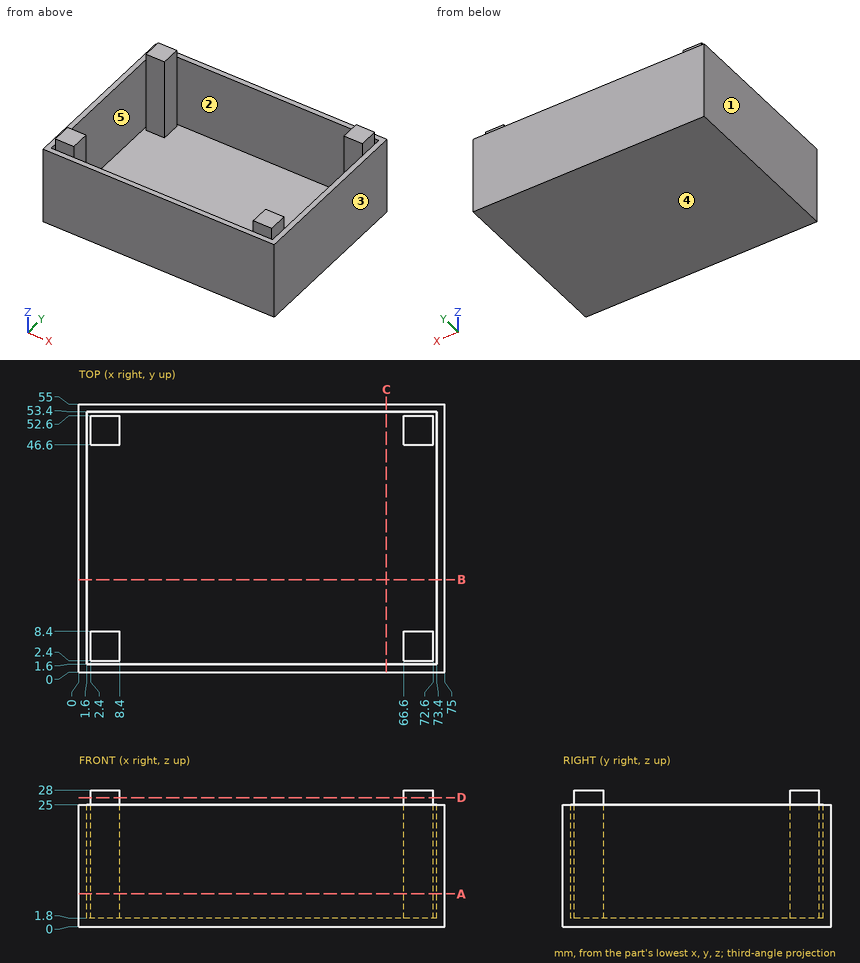
Check sheet for the drawn part. Datum: minimum x, y, z corner. Units: mm. A direction names the side the tool comes from. Give positions to 0.01 mm unless a question says otherwise; leave off trailing zeros. Write each loop counter-clockwise with the first axis right and the second up, starting at its lowest first coordinate (ties: lowest second). Pieces come first, ordered by that corner, then holes. Notation, with made-up numbers: M 54,12.25 L 80,12.25 A19 ccw 80,40.25 Z; hole C 18.25,35 d5. An arc over 180 degrees is marked long. Write item = value, one per line.
(1) Sectioned sample at D-D (z = 26.5). Record the cut outline in (x, y), then the cut area to 3 significant figures.
Found:
outline = M 2.4,2.4 L 8.4,2.4 L 8.4,8.4 L 2.4,8.4 Z; M 2.4,46.6 L 8.4,46.6 L 8.4,52.6 L 2.4,52.6 Z; M 66.6,2.4 L 72.6,2.4 L 72.6,8.4 L 66.6,8.4 Z; M 66.6,46.6 L 72.6,46.6 L 72.6,52.6 L 66.6,52.6 Z
area = 144 mm2
(2) Draft check along X on the marked faces 1, 2 and 3. Enter one of: released by +X, released by -X, zero draft, split by the parting line, or undercut.
Found:
face_1 = released by -X
face_2 = undercut
face_3 = released by +X
(3) Sectioned sample at B-B (y = 19). Record the cut outline in (x, z), then the cut area to 3 significant figures.
Found:
outline = M 0,0 L 75,0 L 75,25 L 73.4,25 L 73.4,1.8 L 1.6,1.8 L 1.6,25 L 0,25 Z
area = 209 mm2
(4) Go/stop test with a flat-tipped pin: pin 1 Ø1 at (x, y) = (67, 40) entering from +Z. Record where the tip stops, or that it passes through.
Found:
pin_1 = 1.8
(5) Material ranges on line 1 (X direction, y = 52, z = 3); line 2 (Y direction, x = 3, z = 18.25); line 3 (Y direction, x = 58.5, z = 16.25), recorded low to high.
Found:
line_1 = 0 to 1.6, 2.4 to 8.4, 66.6 to 72.6, 73.4 to 75
line_2 = 0 to 1.6, 2.4 to 8.4, 46.6 to 52.6, 53.4 to 55
line_3 = 0 to 1.6, 53.4 to 55
(6) Sectioned sample at A-A (z = 6.75). Record the cut outline in (x, y).
Found:
outline = M 0,0 L 75,0 L 75,55 L 0,55 Z; M 2.4,2.4 L 8.4,2.4 L 8.4,8.4 L 2.4,8.4 Z; M 2.4,46.6 L 8.4,46.6 L 8.4,52.6 L 2.4,52.6 Z; M 66.6,2.4 L 72.6,2.4 L 72.6,8.4 L 66.6,8.4 Z; M 66.6,46.6 L 72.6,46.6 L 72.6,52.6 L 66.6,52.6 Z; hole M 1.6,1.6 L 73.4,1.6 L 73.4,53.4 L 1.6,53.4 Z
(7) Access from +Z, -Z, +X, -X, +Y, -Y to the whole of each face (thin tool, end or side, straight path). Record for the marked faces 4 and 5.
Found:
face_4 = -Z, +X, -X, +Y, -Y
face_5 = +Z
(8) Sectioned sample at C-C (x = 63). Record the cut outline in (y, z), then the cut area to 3 significant figures.
Found:
outline = M 0,0 L 55,0 L 55,25 L 53.4,25 L 53.4,1.8 L 1.6,1.8 L 1.6,25 L 0,25 Z
area = 173 mm2
